Source: CAD feature listing. Evaluate the final solid. Frame: model axes, mm. A direction names the side the tool comes from. Coordinates: 2 decimals unless noted, no trailing zeros. Write each loop counter-clockwise with the first axis right and the second up, starting at its lowest first coordinate (ties: lowest second). Pieces come first, ordered by that corner, then holes. Notation, with made-up numbers: (-22, -31.75) - (7, -31.75) arc R7 cw to (7, -22.75) - close; hole circle Ø7 at (-35.75, -20). An arc over 180 degrees is marked (long way). One line per question, with ' | ' between items.
from build123d import *

# Parameters (mm, degrees)
F0_R     = 1.5
F1_DEPTH = 18
F2_R     = 1
F3_DEPTH = 20
F4_DEPTH = 2


with BuildPart() as f1:
    # F0 (on Right) → F1 (new body)
    with BuildSketch(Plane.YZ):
        with BuildLine():
            ThreePointArc((14.8660687473, -2), (14.9664797332, -1.0022396895), (15, 0))
            ThreePointArc((15, 0), (14.9664797332, 1.0022396895), (14.8660687473, 2))
            ThreePointArc((14.8660687473, 2), (10.6066017178, 10.6066017178), (2, 14.8660687473))
            ThreePointArc((2, 14.8660687473), (0, 15), (-2, 14.8660687473))
            ThreePointArc((-2, 14.8660687473), (-10.6066017178, 10.6066017178), (-14.8660687473, 2))
            ThreePointArc((-14.8660687473, 2), (-15, 0), (-14.8660687473, -2))
            ThreePointArc((-14.8660687473, -2), (-10.6066017178, -10.6066017178), (-2, -14.8660687473))
            ThreePointArc((-2, -14.8660687473), (0, -15), (2, -14.8660687473))
            ThreePointArc((2, -14.8660687473), (10.6066017178, -10.6066017178), (14.8660687473, -2))
        make_face()
        with BuildLine():
            ThreePointArc((-2, -11.8321595662), (-8.4852813742, -8.4852813742), (-11.8321595662, -2))
            Line((-11.8321595662, -2), (-2, -2))
            Line((-2, -2), (-2, -11.8321595662))
        make_face(mode=Mode.SUBTRACT)
        Circle(F0_R, mode=Mode.SUBTRACT)
        with BuildLine():
            ThreePointArc((2, 11.8321595662), (8.4852813742, 8.4852813742), (11.8321595662, 2))
            Line((11.8321595662, 2), (2, 2))
            Line((2, 2), (2, 11.8321595662))
        make_face(mode=Mode.SUBTRACT)
    extrude(amount=F1_DEPTH)

    # F2
    f2_edges = [f1.edges().sort_by_distance(p)[0] for p in [
        (0, 14.866069, 2),
        (18, 14.866069, 2),
    ]]
    fillet(f2_edges, radius=F2_R)

    # F0 (on Right) → F3 (join)
    with BuildSketch(Plane.YZ):
        Circle(F0_R)
    extrude(amount=F3_DEPTH)

    # F0 (on Right) → F4 (join)
    with BuildSketch(Plane.YZ):
        Circle(F0_R)
    extrude(amount=-F4_DEPTH)


solid = f1.part
Item 1: Cut plane B-B on y = 0. Return loops of the section in (x, z), and give its area (3 significant figures).
Check sheet entries:
outline: (-2, -1.5) - (0, -1.5) - (0, -14) arc R1 ccw to (1, -15) - (17, -15) arc R1 ccw to (18, -14) - (18, -1.5) - (20, -1.5) - (20, 1.5) - (18, 1.5) - (18, 14) arc R1 ccw to (17, 15) - (1, 15) arc R1 ccw to (0, 14) - (0, 1.5) - (-2, 1.5) - close | area: 551 mm²
Item 2: Access query for faces 4 (the face through (18.99, -1.5, 0.07)), 5 (the face through (9, -2, -7)), 6 (the face through (20, 0, 0)). Directions: +Z, -Z, +X, -X, +Y, -Y. A direction counts if a zero-diameter tool reaches every point of the face in a straight line with its end or side. Return the directions, or none.
Check sheet entries:
face 4: +X | face 5: +X, -X | face 6: +Z, -Z, +X, +Y, -Y
Item 3: Ray query, line 1 along X through (y, z) = (-6.25, 10); line 2 along Z through (x, y) = (16, -9.75); line 3 along Z through (x, y) = (11, -10.5). Return the intervals inside material, ascending. Write a range as [from, to].
Check sheet entries:
line 1: [0, 18] | line 2: [-11.4, -7], [-2, 11.4] | line 3: [-10.71, -5.81], [-2, 10.71]
Item 4: Mould query, pull axis Z, two halves, no side actions, for faces 1 (the face through (0, 3, 0)), 2 (the face through (9, 7, 2)), 3 (the face through (-0.99, -1.5, 0.07)). Classes: pulls with the +Z half, pulls with the -Z half, needs draft (parallel to the pull), parting line crosses it, or undercut.
Check sheet entries:
face 1: needs draft | face 2: undercut | face 3: parting line crosses it
Item 5: Pin query (flat end, axial travel): pin 1 Ø8 at (x, z) = (11.5, 4.5) entering from +Y; pin 2 Ø3 at (y, z) = (-2.5, -11) entering from -X; pin 3 Ø11 at (x, y) = (12.5, 6) entering from +Z. Return the tip coordinate at first contact, or that it passes through.
Check sheet entries:
pin 1: y = 14.99 | pin 2: x = 0 | pin 3: z = 14.99
Item 6: Cut plane A-A on x = 12.5. Return loops of the section in (y, z).
Check sheet entries:
outline: circle Ø30 at (0, 0); hole (-11.83, -2) arc R12 ccw to (-2, -11.83) - (-2, -2) - close; hole (2, 2) - (11.83, 2) arc R12 ccw to (2, 11.83) - close
